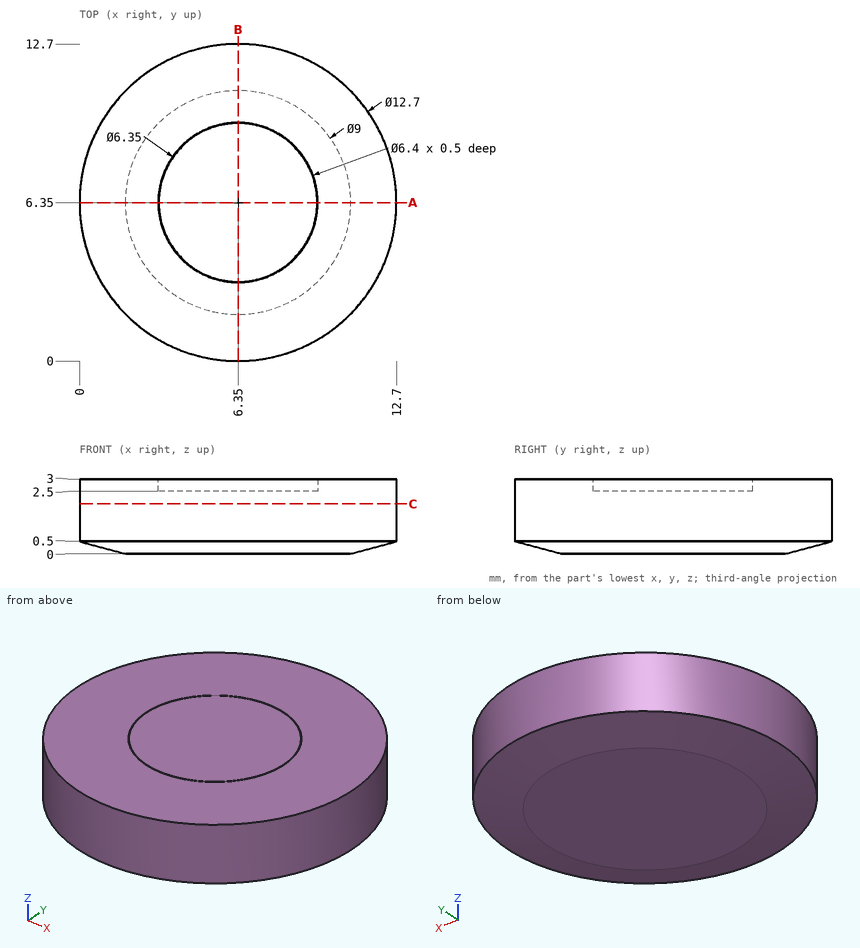
Source: three-view drawing plus pictorial views. Frame: mm from the lowest corner of the part. Coordinates: 2 decimals unless noted, no trailing zeros. Loops run counter-clockwise (first coordinate to the right, second up) from the corner with the lowest first, then second, coordinate; pieces in that order, holes last. Notation, with made-up numbers: (44, 31.5) - (98, 31.5) arc R11 ccw to (98, 35.5) - close; hole circle Ø10 at (40, 42.25). An arc over 180 degrees is marked (long way). One line per question, with ' | ' between items.
1) Section A-A, the plane y = 6.35. Return loops of the section in (x, z) (3 decimals).
Report:
outline: (0, 0.5) - (1.85, 0) - (10.85, 0) - (12.7, 0.5) - (12.7, 3) - (9.55, 3) - (9.55, 2.5) - (9.525, 2.5) - (9.525, 3) - (3.175, 3) - (3.175, 2.5) - (3.15, 2.5) - (3.15, 3) - (0, 3) - close
2) Line query: line 1 along Z through (x, y) = (8.25, 11.75); line 2 along Y through (x, z) = (10, 2.2); line 3 along Z through (x, y) = (7, 12.25). Output: solid intervals per line, ascending.
Report:
line 1: z = 0.33 to 3 | line 2: y = 1.15 to 11.55 | line 3: z = 0.39 to 3
3) Section C-C, the plane z = 2. Return loops of the section in (x, y), then the cut area to 3 significant figures.
Report:
outline: circle Ø12.7 at (6.35, 6.35) | area: 127 mm²
4) First-contact query: P1, Ø1, axis at x = 1.5, z = 0.5, coming from the +Y side; P2, Ø1, axis at x = 2.5, y = 4, coming from the -Z side; P3, Ø1, axis at x = 9.5, z = 1, coming from the -Y side; P4, Ø1, axis at y = 2, z = 2.5, coming from the +X side. Flat tips, straight axial feed; report the tip coordinate or a pass-through.
Report:
P1: stops at y = 10.98 | P2: stops at z = 0 | P3: stops at y = 0.58 | P4: stops at x = 11.4
